from build123d import *

# Parameters (mm, degrees)
BOSS_EXTRUDE1_DEPTH       = 10
SKETCH2_W                 = 7
SKETCH2_H                 = 54
BOSS_EXTRUDE2_DEPTH       = 15.494
SKETCH3_W                 = 7
SKETCH3_H                 = 54
BOSS_EXTRUDE3_DEPTH       = 34
SKETCH5_R                 = 11
CUT_EXTRUDE2_DEPTH        = 4
SKETCH6_R                 = 4
CUT_EXTRUDE3_DEPTH        = 10
SKETCH7_W                 = 34
SKETCH7_H                 = 7
BOSS_EXTRUDE4_DEPTH       = 25
BOSS_EXTRUDE5_DEPTH       = 32
F_3_0MM_DOWEL_HOLE1_D     = 3
F_3_0MM_DOWEL_HOLE1_DEPTH = 27
F_3_0MM_DOWEL_HOLE1_TIP   = 0.901290929
FILLET2_R                 = 5
FILLET3_R                 = 5


with BuildPart() as part:
    # Sketch1 → Boss-Extrude1 (new body)
    with BuildSketch(Plane.XY):
        Polygon((0, 0), (27, 0), (27, 7), (7, 7), (7, 47), (27, 47), (27, 54), (0, 54), align=None)
    extrude(amount=BOSS_EXTRUDE1_DEPTH)

    # Sketch2 → Boss-Extrude2 (add)
    with BuildSketch(Plane(origin=(0, 0, 0), x_dir=(-1, 0, 0), z_dir=(0, 0, -1))):
        with Locations((-3.5, 27)):
            Rectangle(SKETCH2_W, SKETCH2_H)
    extrude(amount=BOSS_EXTRUDE2_DEPTH)

    # Sketch3 → Boss-Extrude3 (add)
    with BuildSketch(Plane.ZY):
        with Locations((-18.994, 27)):
            Rectangle(SKETCH3_W, SKETCH3_H)
    extrude(amount=-BOSS_EXTRUDE3_DEPTH)

    # Sketch5 → Cut-Extrude2 (cut)
    with BuildSketch(Plane(origin=(0, 0, -22.494), x_dir=(-1, 0, 0), z_dir=(0, 0, -1))):
        with Locations(Location((-17.1, 37.04, 0), (0, 0, 90))):
            Circle(SKETCH5_R)
    extrude(amount=-CUT_EXTRUDE2_DEPTH, mode=Mode.SUBTRACT)

    # Sketch6 → Cut-Extrude3 (cut)
    with BuildSketch(Plane(origin=(0, 0, -18.494), x_dir=(-1, 0, 0), z_dir=(0, 0, -1))):
        with Locations(Location((-17.1, 37.04, 0), (0, 0, 90))):
            Circle(SKETCH6_R)
    extrude(amount=-CUT_EXTRUDE3_DEPTH, mode=Mode.SUBTRACT)

    # Sketch7 → Boss-Extrude4 (add)
    with BuildSketch(Plane.XZ):
        with Locations((17, -18.994)):
            Rectangle(SKETCH7_W, SKETCH7_H)
    extrude(amount=BOSS_EXTRUDE4_DEPTH)

    # Sketch8 → Boss-Extrude5 (add)
    with BuildSketch(Plane.XZ.offset(25)):
        Polygon((0, -22.494), (0, -30.494), (34, -30.494), (34, -26.494), (7, -26.494), (7, -22.494), align=None)
    extrude(amount=-BOSS_EXTRUDE5_DEPTH)

    # Ø3.0mm Dowel Hole1
    with Locations(Plane(origin=(0, 0, -30.494), x_dir=(-1, 0, 0), z_dir=(0, 0, -1))):
        with Locations((-22.1, -10), (-22.1, 0), (-12.1, 0), (-12.1, -10)):
            Hole(F_3_0MM_DOWEL_HOLE1_D / 2, depth=F_3_0MM_DOWEL_HOLE1_DEPTH)
            with Locations((0, 0, -(F_3_0MM_DOWEL_HOLE1_DEPTH + F_3_0MM_DOWEL_HOLE1_TIP / 2))):  # 118° drill point
                Cone(0, F_3_0MM_DOWEL_HOLE1_D / 2, F_3_0MM_DOWEL_HOLE1_TIP, mode=Mode.SUBTRACT)

    # Fillet2
    fillet2_edges = [part.edges().sort_by_distance(p)[0] for p in [
        (34, -25, -18.994),
        (34, -25, -28.494),
    ]]
    fillet(fillet2_edges, radius=FILLET2_R)

    # Fillet3
    fillet3_edges = [part.edges().sort_by_distance(p)[0] for p in [
        (0, -25, -22.994),
    ]]
    fillet(fillet3_edges, radius=FILLET3_R)


solid = part.part
Read the model definition and answer for the solid it produces. Units are mm, in the model's axes. A direction names the side the tool comes from. Round coordinates to 2 decimals unless told otherwise and drop trailing zeros. Order: outer loops, then holes, each group sorted by start corner. A loop starts at its lowest first (then second) coordinate and runs counter-clockwise, first axis right, second up.
1) For faces 4 (the face through (20.6, 0.07, -18.94)), 5 (the face through (17, 4, 0)), 6 (the face through (27, 3, 5)), determine the directions among +Z, -Z, +X, -X, +Y, -Y from which every point of the face is accessible in a straight line to the end or side of a thin tool.
2) The part is cut by section B-B on x = 17.1. Write down the section's boundary in (y, z), plus the area to 3 significant figures.
3) The part is cut by section A-A on y = -10. Write down the section's boundary in (x, z).
4) Flat-ended cylindrical pins translate along their axes: pin 1 (12.5 mm diameter, centred on x = 16.5, z = -4, fed in from -Y); pin 2 (10 mm diameter, centred on x = 21.5, y = -12.5, fed in from +Z); pin 3 (7.5 mm diameter, centred on y = 4.5, z = 4.5, fed in from +X). Find the tip coordinate at first contact, or state that the pin passes through.
5) Straight lines are drawn through the part: L1, parallel to Z at x = 17.5, y = 6; L2, parallel to Z at x = 20, y = 50.5; L3, parallel to Z at x = 16, y = 47.5. For each, find the intervals that lie inside material, in ascending order.
6) The mould has two halves that part along Y. Classify faces 1 (the face through (17, 15, -22.494)), 2 (the face through (20.6, 0.07, -28.47)), 3 (the face through (32, -24, -28)): released by +Y, released by -Y, zero draft, split by the parting line, or undercut.
7) The part is cut by section C-C on z = -20. Write down the section's boundary in (x, y).
8) The part is cut by section D-D on y = 37.04. Write down the section's boundary in (x, z).
Resolved:
1. face 4: -Z
1. face 5: +X, +Y, -Y
1. face 6: +Z, +X, +Y, -Y
2. outline: (-25, -30.49) - (7, -30.49) - (7, -26.49) - (-25, -26.49) - close; (-25, -22.49) - (26.04, -22.49) - (26.04, -18.49) - (33.04, -18.49) - (33.04, -15.49) - (-25, -15.49) - close; (0, 0) - (7, 0) - (7, 10) - (0, 10) - close; (41.04, -18.49) - (48.04, -18.49) - (48.04, -22.49) - (54, -22.49) - (54, -15.49) - (41.04, -15.49) - close; (47, 0) - (54, 0) - (54, 10) - (47, 10) - close
2. area: 709 mm2
3. outline: (0, -30.49) - (10.6, -30.49) - (10.6, -26.49) - (7, -26.49) - (7, -22.49) - (10.6, -22.49) - (10.6, -15.49) - (0, -15.49) - close; (13.6, -30.49) - (20.6, -30.49) - (20.6, -26.49) - (13.6, -26.49) - close; (13.6, -22.49) - (20.6, -22.49) - (20.6, -15.49) - (13.6, -15.49) - close; (23.6, -30.49) - (34, -30.49) - (34, -26.49) - (23.6, -26.49) - close; (23.6, -22.49) - (34, -22.49) - (34, -15.49) - (23.6, -15.49) - close
4. pin 1: stops at y = 0
4. pin 2: stops at z = -15.49
4. pin 3: stops at x = 27
5. L1: z = -30.49 to -26.49, -22.49 to -15.49, 0 to 10
5. L2: z = -22.49 to -15.49, 0 to 10
5. L3: z = -18.49 to -15.49, 0 to 10
6. face 1: zero draft
6. face 2: undercut
6. face 3: released by -Y
7. outline: (0, -20) arc R5 ccw to (5, -25) - (29, -25) arc R5 ccw to (34, -20) - (34, 54) - (0, 54) - close; hole circle Ø22 at (17.1, 37.04); hole circle Ø3 at (12.1, -10); hole circle Ø3 at (12.1, 0); hole circle Ø3 at (22.1, -10); hole circle Ø3 at (22.1, 0)
8. outline: (0, -22.49) - (6.1, -22.49) - (6.1, -18.49) - (13.1, -18.49) - (13.1, -15.49) - (7, -15.49) - (7, 10) - (0, 10) - close; (21.1, -18.49) - (28.1, -18.49) - (28.1, -22.49) - (34, -22.49) - (34, -15.49) - (21.1, -15.49) - close
